Read the model definition and answer for the solid it produces. Units are mm, in the model's axes. Face numbers are marked on the shaded views. A direction names the side the tool comes from. Give positions to 0.01 mm unless a question says otherwise; leave off trailing zeros. Loops run counter-clockwise (first coordinate to the right, second up) from the corner with the lowest first, then second, coordinate; pieces in that order, holes last. Notation, with made-up numbers: (-4, -17.5) - (28, -17.5) arc R17 ccw to (28, -11.5) - close; hole circle Ø10 at (3.25, 4). An arc over 180 degrees is marked (long way). Use a Markdown table: item, result. Add a question column.
Item 1: A cutting plane is placed at B-B (x = 0). Give the number of separate pieces and of enclosed holes in the cut face, plus the area to 3 significant figures.
Item 2: For a pull along X with two mould halves and no side action, classify the marked faces 1, 2 and 3 as +X half, -X half, draft (parallel to the pull), parting line (faces both ways), or undercut.
Item 3: Which of the six approach directions +Z, -Z, +X, -X, +Y, -Y give full straight-line access (tool end or side, diameter ignored) to the marked faces 4 and 5?
Item 4: A cutting plane is placed at A-A (y = -57.25). Determine the outline of the cut face in (x, z), plus the area to 3 significant figures.
Item 5: Consider probe 1 along Y at (x, z) = (0, 73); probe 2 along X at (y, z) = (-74.75, 72.05); probe 3 along X at (y, z) = (-108, 74.25). Determine where each line is inside the solid, lowest interval first. Write a range as [from, to].
Item 6: Each of these flat-tipped pins is pushed along its axis until it touches: P1, Ø6, axis at y = -77.5, z = 72.5, coming from the +X side; P2, Ø3.5, axis at x = 0, y = -127.25, coming from the +Z side; P3, Ø1.5, axis at y = -81.5, z = 73, coming from the -X side; P4, Ø2.5, axis at x = 0, y = -57.25, coming from the -Z side. Where does it stop, or does it pass through?
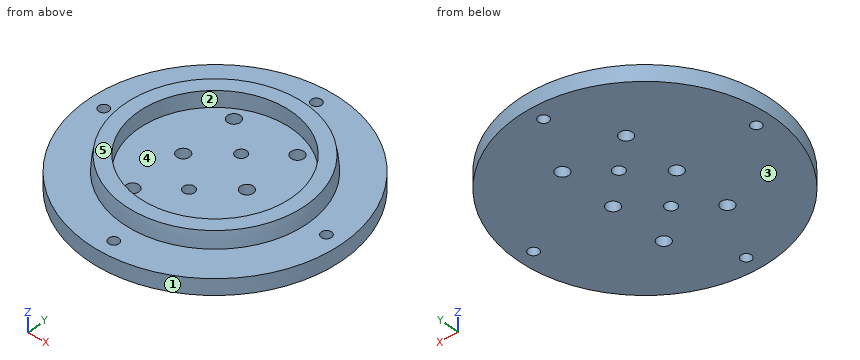
from build123d import *

# Parameters (mm, degrees)
CYLINDER089_R     = 1.6
CYLINDER089_DEPTH = 10
CYLINDER090_R     = 1.6
CYLINDER090_DEPTH = 10
CYLINDER091_R     = 1.6
CYLINDER091_DEPTH = 10
CYLINDER088_R     = 1.6
CYLINDER088_DEPTH = 10
CYLINDER085_R     = 2
CYLINDER085_DEPTH = 10
CYLINDER084_R     = 2
CYLINDER084_DEPTH = 10
CYLINDER087_R     = 1.75
CYLINDER087_DEPTH = 10
CYLINDER086_R     = 1.75
CYLINDER086_DEPTH = 10
CYLINDER078_R     = 2
CYLINDER078_DEPTH = 10
CYLINDER079_R     = 2
CYLINDER079_DEPTH = 10
CYLINDER080_R     = 2
CYLINDER080_DEPTH = 10
CYLINDER081_R     = 2
CYLINDER081_DEPTH = 10
CYLINDER083_R     = 24
CYLINDER083_DEPTH = 7
CYLINDER082_R     = 40
CYLINDER082_DEPTH = 5


with BuildPart() as obj1:
    # Cylinder089 → Cylinder089 (new body)
    with BuildSketch(Plane(origin=(40, 0, 65), x_dir=(1, 0, 0), z_dir=(0, 0, 1))):
        Circle(CYLINDER089_R)
    extrude(amount=CYLINDER089_DEPTH)


with BuildPart() as obj2:
    # Cylinder090 → Cylinder090 (new body)
    with BuildSketch(Plane(origin=(5, 35, 65), x_dir=(1, 0, 0), z_dir=(0, 0, 1))):
        Circle(CYLINDER090_R)
    extrude(amount=CYLINDER090_DEPTH)


with BuildPart() as obj3:
    # Cylinder091 → Cylinder091 (new body)
    with BuildSketch(Plane(origin=(5, -35, 65), x_dir=(1, 0, 0), z_dir=(0, 0, 1))):
        Circle(CYLINDER091_R)
    extrude(amount=CYLINDER091_DEPTH)


with BuildPart() as fusion045:
    # Cylinder088 → Cylinder088 (new body)
    with BuildSketch(Plane(origin=(-30, 0, 65), x_dir=(1, 0, 0), z_dir=(0, 0, 1))):
        Circle(CYLINDER088_R)
    extrude(amount=CYLINDER088_DEPTH)

    # Fusion045: union obj1, obj2, obj3
    add(obj1.part)
    add(obj2.part)
    add(obj3.part)


with BuildPart() as wirecut009:
    # Cylinder085 → Cylinder085 (new body)
    with BuildSketch(Plane(origin=(15, 0, 70), x_dir=(1, 0, 0), z_dir=(0, 0, 1))):
        Circle(CYLINDER085_R)
    extrude(amount=CYLINDER085_DEPTH)


with BuildPart() as wirecuts004:
    # Cylinder084 → Cylinder084 (new body)
    with BuildSketch(Plane(origin=(-5, 0, 70), x_dir=(1, 0, 0), z_dir=(0, 0, 1))):
        Circle(CYLINDER084_R)
    extrude(amount=CYLINDER084_DEPTH)

    # Fusion041: union wireCUt009
    add(wirecut009.part)


with BuildPart() as m3cuts009:
    # Cylinder087 → Cylinder087 (new body)
    with BuildSketch(Plane(origin=(5, 9, 70), x_dir=(1, 0, 0), z_dir=(0, 0, 1))):
        Circle(CYLINDER087_R)
    extrude(amount=CYLINDER087_DEPTH)


with BuildPart() as m3cute004:
    # Cylinder086 → Cylinder086 (new body)
    with BuildSketch(Plane(origin=(5, -9, 70), x_dir=(1, 0, 0), z_dir=(0, 0, 1))):
        Circle(CYLINDER086_R)
    extrude(amount=CYLINDER086_DEPTH)

    # Fusion042: union m3Cuts009
    add(m3cuts009.part)


with BuildPart() as cylinder078:
    # Cylinder078 → Cylinder078 (new body)
    with BuildSketch(Plane(origin=(0, -21, 0), x_dir=(1, 0, 0), z_dir=(0, 0, 1))):
        Circle(CYLINDER078_R)
    extrude(amount=CYLINDER078_DEPTH)


with BuildPart() as m3heatsetcuts012:
    # Cylinder079 → Cylinder079 (new body)
    with BuildSketch(Plane(origin=(20, -21, 0), x_dir=(1, 0, 0), z_dir=(0, 0, 1))):
        Circle(CYLINDER079_R)
    extrude(amount=CYLINDER079_DEPTH)

    # Fusion038: union Cylinder078
    add(cylinder078.part)


with BuildPart() as m3heatsetcuts012_1:
    # Fusion038 placement: moved
    add(m3heatsetcuts012.part.moved(Location((-5, 38.5, 70))))


with BuildPart() as cylinder080:
    # Cylinder080 → Cylinder080 (new body)
    with BuildSketch(Plane(origin=(0, -21, 0), x_dir=(1, 0, 0), z_dir=(0, 0, 1))):
        Circle(CYLINDER080_R)
    extrude(amount=CYLINDER080_DEPTH)


with BuildPart() as basecuts004:
    # Cylinder081 → Cylinder081 (new body)
    with BuildSketch(Plane(origin=(20, -21, 0), x_dir=(1, 0, 0), z_dir=(0, 0, 1))):
        Circle(CYLINDER081_R)
    extrude(amount=CYLINDER081_DEPTH)

    # Fusion039: union Cylinder080
    add(cylinder080.part)


with BuildPart() as basecuts004_1:
    # Fusion039 placement: moved
    add(basecuts004.part.moved(Location((-5, 3.5, 70))))

    # Fusion040: union m3HeatSetCuts012
    add(m3heatsetcuts012_1.part)

    # Fusion043: union wireCuts004, m3Cute004
    add(wirecuts004.part)
    add(m3cute004.part)


with BuildPart() as basecut004:
    # Cylinder083 → Cylinder083 (new body)
    with BuildSketch(Plane(origin=(5, 0, 74), x_dir=(1, 0, 0), z_dir=(0, 0, 1))):
        Circle(CYLINDER083_R)
    extrude(amount=CYLINDER083_DEPTH)


with BuildPart() as cut015:
    # Sphere005 → Sphere005 (revolve)
    with BuildSketch(Plane(origin=(5, 0, 74), x_dir=(1, 0, 0), z_dir=(0, -1, 0))):
        with BuildLine():
            ThreePointArc((29, 0), (28.841135, 3.031325), (28.36628, 6.029439))
            Line((28.36628, 6.029439), (0, 6.029439))
            Line((0, 6.029439), (0, 0))
            Line((0, 0), (29, 0))
        make_face()
    revolve(axis=Axis((5, 0, 74), (0, 0, 1)))

    # Cut015: cut baseCut004
    add(basecut004.part, mode=Mode.SUBTRACT)


with BuildPart() as lightmodule004:
    # Cylinder082 → Cylinder082 (new body)
    with BuildSketch(Plane(origin=(5, 0, 70), x_dir=(1, 0, 0), z_dir=(0, 0, 1))):
        Circle(CYLINDER082_R)
    extrude(amount=CYLINDER082_DEPTH)

    # Fusion044: union Cut015
    add(cut015.part)

    # Cut016: cut baseCUts004
    add(basecuts004_1.part, mode=Mode.SUBTRACT)

    # Cut017: cut Fusion045
    add(fusion045.part, mode=Mode.SUBTRACT)


with BuildPart() as lightmodule004_1:
    # Cut017 placement: moved
    add(lightmodule004.part.moved(Location((-5, -92.25, 0))))


solid = lightmodule004_1.part
Geometry says:
| question | item | result |
|---|---|---|
| 1 | separate pieces | 5 |
| 1 | enclosed holes | 0 |
| 1 | area | 381 mm² |
| 2 | face 1 | parting line |
| 2 | face 2 | undercut |
| 2 | face 3 | draft |
| 3 | face 4 | +Z |
| 3 | face 5 | +Z, +X, -X, +Y, -Y |
| 4 | outline | (-19.36, 70) - (-1.6, 70) - (-1.6, 75) - (-19.36, 75) - close; (1.6, 70) - (19.36, 70) - (19.36, 75) - (1.6, 75) - close |
| 4 | area | 178 mm² |
| 5 | probe 1 | [-132.25, -128.85], [-125.65, -103], [-99.5, -85], [-81.5, -58.85], [-55.65, -52.25] |
| 5 | probe 2 | [-35.97, -12], [-8, 8], [12, 35.97] |
| 5 | probe 3 | [-36.77, -10.97], [-9.03, 9.03], [10.97, 36.77] |
| 6 | P1 | x = 38.24 |
| 6 | P2 | z = 75 |
| 6 | P3 | x = -38.73 |
| 6 | P4 | through |
